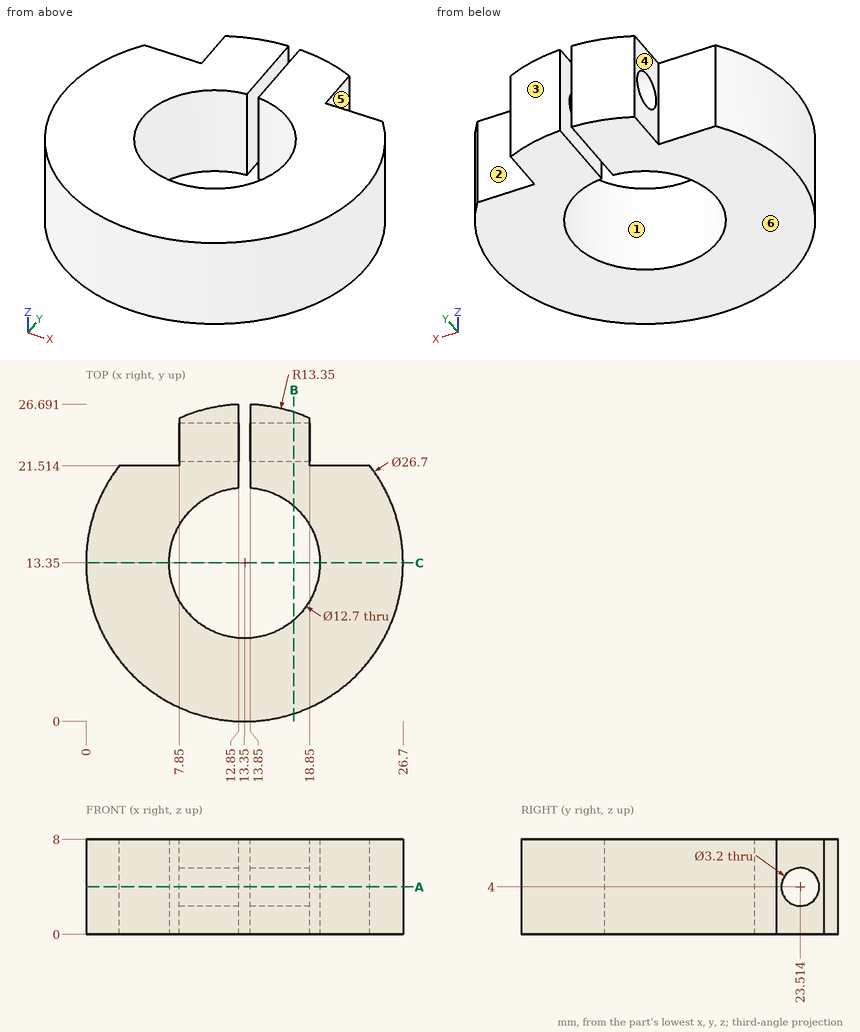
Source: three-view drawing plus pictorial views. Frame: mm from the lowest corner of the part. A direction names the side the tool comes from. Give positions to 0.01 mm unless a question says otherwise; leave off trailing zeros. Order: outer loops, then holes, each group sorted by start corner. A loop starts at its lowest first (then second) coordinate and runs counter-clockwise, first axis right, second up. Notation, with made-up numbers: (-4.5, 41) - (52.5, 41) arc R30 ccw to (52.5, 78) - close; hole circle Ø3 at (22.5, -4.75). An arc over 180 degrees is marked (long way). Answer as a JSON object with one key per item and string values. Group by question number.
Q1. First-contact query: pin 1 Ø2.5 at (x, z) = (22, 3.5) entering from +Y; pin 2 Ø2 at (y, z) = (23, 3) entering from -X; pin 3 Ø3 at (y, z) = (23.51, 4) entering from -X; pin 4 Ø2 at (y, z) = (6.5, 3) entering from +X. Flat tips, straight axial feed; report the tip coordinate or a pass-through.
Q2. Cut plane C-C, the plane y = 13.35. Output: boundary loops of the cut face in (x, z).
Q3. Cut plane A-A, the plane z = 4. Count the separate pieces of the cut face and the enclosed holes in it.
Q4. Cut plane B-B, the plane x = 17.5. Output: boundary loops of the cut face in (y, z) (1 decimal), then the cut area to 3 significant figures.
Q5. Mould query, pull axis X, two halves, no side actions, for the marked faces 1, 2 and 3. Classes: pulls with the +X half, pulls with the -X half, needs draft (parallel to the pull), parting line crosses it, or undercut.
Q6. Line query: probe 1 along X at (y, z) = (13.35, 5.5); probe 2 along X at (y, z) = (21.75, 5); probe 3 along Y at (x, z) = (13.35, 2.25). Output: solid intervals per line, ascending.
Q7. Set-up query: the marked faces 4, 5 and 6. Return all of +Z, -Z, +X, -X, +Y, -Y with unobstructed straight access to the full face (end or side cutting, diameter ignored); none if empty.
Results:
{
 "1": {"pin 1": "y = 21.51", "pin 2": "x = 7.85", "pin 3": "through", "pin 4": "x = 25.35"},
 "2": {"outline": "(0, 0) - (7, 0) - (7, 8) - (0, 8) - close; (19.7, 0) - (26.7, 0) - (26.7, 8) - (19.7, 8) - close"},
 "3": {"separate pieces": "3", "enclosed holes": "0"},
 "4": {"outline": "(0.7, 0) - (8.5, 0) - (8.5, 8) - (0.7, 8) - close; (18.2, 0) - (26, 0) - (26, 8) - (18.2, 8) - close; hole circle Ø3.2 at (23.5, 4)", "area": "118 mm^2"},
 "5": {"face 1": "undercut", "face 2": "needs draft", "face 3": "pulls with the +X half"},
 "6": {"probe 1": "0 to 7, 19.7 to 26.7", "probe 2": "7.85 to 12.85, 13.85 to 18.85", "probe 3": "0 to 7"},
 "7": {"face 4": "+Z, -Z, -X, +Y", "face 5": "+Z, -Z, +X, +Y", "face 6": "-Z, +X, -X, +Y, -Y"}
}
